Can you work these out from the model? Positions are in its coordinate system, mm. Face numbers are marked on the shaded views. A direction names the side the tool comes from. Round coordinates to 2 decimals unless told otherwise and drop trailing zeros. Loops run counter-clockwise (first coordinate to the right, second up) from the corner with the lowest first, then second, coordinate; pieces in that order, holes last. Notation, with made-up numbers: (44.25, 13) -> (67.25, 13) arc R26 cw to (67.25, 27) -> close; hole circle Ø1 at (8.25, -4). An arc over 180 degrees is marked (long way). Answer as a JSON object with one key per item and string values.
```python
from build123d import *

# Parameters (mm, degrees)
BOSS_EXTRUDE1_DEPTH = 50
SKETCH2_W           = 5
SKETCH2_H           = 26.35
BOSS_EXTRUDE2_DEPTH = 20
SKETCH4_W           = 5
SKETCH4_H           = 26.35
BOSS_EXTRUDE3_DEPTH = 20
FILLET2_R           = 2


with BuildPart() as part:
    # Sketch1 → Boss-Extrude1 (new body)
    with BuildSketch(Plane.XY):
        Polygon((27.292868212, 8.549060403), (-35.507131788, 8.549060403), (-35.507131788, -17.800939597), (-15.507131788, -17.800939597), (-15.507131788, -7.800939597), (-30.507131788, -7.800939597), (-30.507131788, -1.450939597), (22.292868212, -1.450939597), (22.292868212, -7.800939597), (7.292868212, -7.800939597), (7.292868212, -17.800939597), (27.292868212, -17.800939597), align=None)
    extrude(amount=-BOSS_EXTRUDE1_DEPTH)

    # Sketch2 → Boss-Extrude2 (add)
    with BuildSketch(Plane.XY):
        with Locations((-33.007131788, -4.625939597)):
            Rectangle(SKETCH2_W, SKETCH2_H)
        with Locations((24.792868212, -4.625939597)):
            Rectangle(SKETCH2_W, SKETCH2_H)
    extrude(amount=BOSS_EXTRUDE2_DEPTH)

    # Sketch4 → Boss-Extrude3 (add)
    with BuildSketch(Plane(origin=(0, 0, -50), x_dir=(-1, 0, 0), z_dir=(0, 0, -1))):
        with Locations((-24.792868212, -4.625939597)):
            Rectangle(SKETCH4_W, SKETCH4_H)
        with Locations((33.007131788, -4.625939597)):
            Rectangle(SKETCH4_W, SKETCH4_H)
    extrude(amount=BOSS_EXTRUDE3_DEPTH)

    # Fillet2
    fillet2_edges = [part.edges().sort_by_distance(p)[0] for p in [
        (-15.507131788, -12.800939597, -50),
        (14.792868212, -17.800939597, 0),
        (7.292868212, -12.800939597, 0),
        (-15.507131788, -12.800939597, 0),
        (7.292868212, -17.800939597, -25),
        (-15.507131788, -17.800939597, -25),
        (-23.007131788, -17.800939597, 0),
        (-30.507131788, -12.800939597, 0),
        (7.292868212, -12.800939597, -50),
        (-30.507131788, 8.549060403, 10),
        (-30.507131788, -17.800939597, 10),
        (-30.507131788, 3.549060403, 0),
        (14.792868212, -17.800939597, -50),
        (-4.107131788, 8.549060403, 0),
        (22.292868212, 3.549060403, 0),
        (22.292868212, -12.800939597, 0),
        (22.292868212, 8.549060403, 10),
        (22.292868212, -17.800939597, 10),
        (-4.107131788, 8.549060403, -50),
        (22.292868212, 3.549060403, -50),
        (22.292868212, -12.800939597, -50),
        (22.292868212, -17.800939597, -60),
        (22.292868212, 8.549060403, -60),
        (-23.007131788, -17.800939597, -50),
        (-30.507131788, 3.549060403, -50),
        (-30.507131788, -12.800939597, -50),
        (-30.507131788, 8.549060403, -60),
        (-30.507131788, -17.800939597, -60),
    ]]
    fillet(fillet2_edges, radius=FILLET2_R)


solid = part.part
```
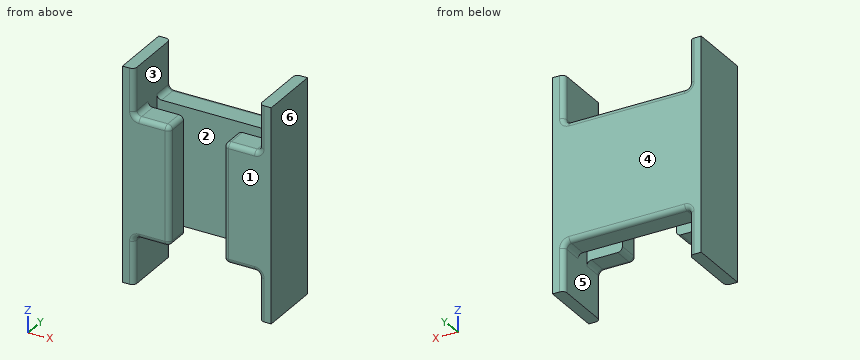
Q1. If I drill on L1, parallel to Y at x = 15, z = -14.5; L2, parallel to X at y = 5, z = 8.5; L3, parallel to Z at x = -9, y = 4.25, over which ranges is the centre line in solid material (lowest first)? Write a range as [from, to].
Determined:
{"L1": "[-17.8, -7.8], [-1.45, 8.55]", "L2": "[-35.51, -30.51], [22.29, 27.29]", "L3": "[-50, 0]"}
Q2. I want a section at C-C, the plane x = -21.5. Write out the boundary of the cut face in (y, z).
Determined:
{"outline": "(-17.8, -48) arc R2 ccw to (-15.8, -50) -> (-7.8, -50) -> (-7.8, 0) -> (-15.8, 0) arc R2 ccw to (-17.8, -2) -> close; (-1.45, -50) -> (6.55, -50) arc R2 ccw to (8.55, -48) -> (8.55, -2) arc R2 ccw to (6.55, 0) -> (-1.45, 0) -> close"}
Q3. I want a section at B-B, the plane z = 4. Write out the boundary of the cut face in (x, y), then the cut area to 3 significant figures.
Determined:
{"outline": "(-35.51, -17.8) -> (-32.51, -17.8) arc R2 ccw to (-30.51, -15.8) -> (-30.51, 6.55) arc R2 ccw to (-32.51, 8.55) -> (-35.51, 8.55) -> close; (22.29, -15.8) arc R2 ccw to (24.29, -17.8) -> (27.29, -17.8) -> (27.29, 8.55) -> (24.29, 8.55) arc R2 ccw to (22.29, 6.55) -> close", "area": "260 mm²"}
Q4. On a 3-axis mill with a long thin cutter (end or side, diameter ignored), from which of +Z, -Z, +X, -X, +Y, -Y can I reach the whole of each face in a straight line? I mean the marked faces 1 and 2. Say none if no direction works.
Determined:
{"face 1": "+Z, -Z, +X, -X, -Y", "face 2": "+Z, -Z"}
Q5. I want a section at A-A, the plane y = -3.25. Write out the boundary of the cut face in (x, z), then the cut area to 3 significant figures.
Determined:
{"outline": "(-35.51, -70) -> (-30.51, -70) -> (-30.51, 20) -> (-35.51, 20) -> close; (22.29, -70) -> (27.29, -70) -> (27.29, 20) -> (22.29, 20) -> close", "area": "900 mm²"}
Q6. I want a section at D-D, the plane z = -41. Write out the boundary of the cut face in (x, y), then the cut area to 3 significant figures.
Determined:
{"outline": "(-35.51, -17.8) -> (-17.51, -17.8) arc R2 ccw to (-15.51, -15.8) -> (-15.51, -7.8) -> (-30.51, -7.8) -> (-30.51, -1.45) -> (22.29, -1.45) -> (22.29, -7.8) -> (7.29, -7.8) -> (7.29, -15.8) arc R2 ccw to (9.29, -17.8) -> (27.29, -17.8) -> (27.29, 8.55) -> (-35.51, 8.55) -> close", "area": "1,090 mm²"}
Q7. We'd pull the mould along Y, two halves only. Please class the marked faces 3, 4, 5 and 6: pulls with the +Y half, pulls with the -Y half, needs draft (parallel to the pull), parting line crosses it, or undercut.
Determined:
{"face 3": "undercut", "face 4": "pulls with the +Y half", "face 5": "undercut", "face 6": "needs draft"}
Q8. I'm going to push flat-ended pins straight in: pin 1 (4 mm diameter, centred on x = 16.5, y = -10, fed in from +Z); pin 2 (4 mm diameter, centred on x = -15, y = 1.5, fed in from -Z). Where does each tip first touch, or does it pass through?
Determined:
{"pin 1": "z = 0", "pin 2": "z = -50"}
